Source: CAD feature listing. Evaluate the final solid. Frame: model axes, mm. Face numbers are marked on the shaded views. A direction names the side the tool comes from. Round coordinates to 2 decimals unless told otherwise and drop trailing zeros. Order: outer loops, then holes, each group sorted by start corner. A loop starts at its lowest first (then second) coordinate and runs counter-clockwise, first axis right, second up.
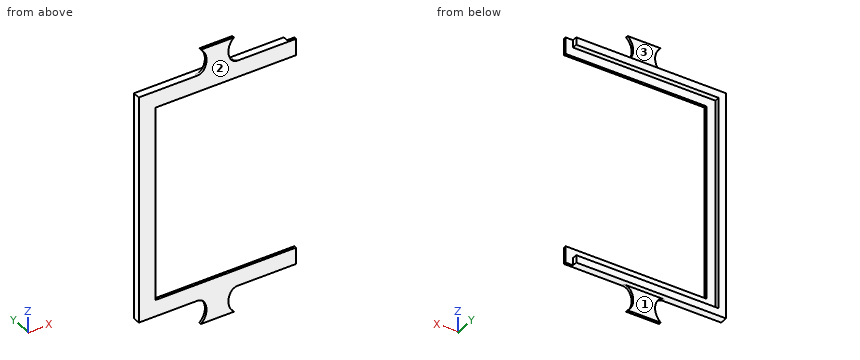
```python
from build123d import *

# Parameters (mm, degrees)
SKETCH1_W           = 10
SKETCH1_H           = 117.5
BOSS_EXTRUDE1_DEPTH = 1.5
BOSS_EXTRUDE2_DEPTH = 3


with BuildPart() as part:
    # Sketch1 → Boss-Extrude1 (new body)
    with BuildSketch(Plane(origin=(0, 0, 0), x_dir=(1, 0, 0), z_dir=(0, 1, 0))):
        with BuildLine():
            ThreePointArc((-7.95412424, -71.25), (-9.784251259, -69.419872981), (-12.284251259, -68.75))
            Line((-12.284251259, -68.75), (-47.65, -68.75))
            Line((-47.65, -68.75), (-47.65, -58.75))
            Line((-47.65, -58.75), (47.65, -58.75))
            Line((47.65, -58.75), (47.65, -68.75))
            Line((47.65, -68.75), (12.284251259, -68.75))
            ThreePointArc((12.284251259, -68.75), (9.784251259, -69.419872981), (7.95412424, -71.25))
            ThreePointArc((7.95412424, -71.25), (6.745685452, -77.865209555), (10, -83.75))
            Line((10, -83.75), (-10, -83.75))
            ThreePointArc((-10, -83.75), (-6.745685452, -77.865209555), (-7.95412424, -71.25))
        make_face()
        with Locations((-42.65, 0)):
            Rectangle(SKETCH1_W, SKETCH1_H)
        with BuildLine():
            ThreePointArc((-7.95412424, 71.25), (-6.745685452, 77.865209555), (-10, 83.75))
            Line((-10, 83.75), (10, 83.75))
            ThreePointArc((10, 83.75), (6.745685452, 77.865209555), (7.95412424, 71.25))
            ThreePointArc((7.95412424, 71.25), (9.784251259, 69.419872981), (12.284251259, 68.75))
            Line((12.284251259, 68.75), (47.65, 68.75))
            Line((47.65, 68.75), (47.65, 58.75))
            Line((47.65, 58.75), (-47.65, 58.75))
            Line((-47.65, 58.75), (-47.65, 68.75))
            Line((-47.65, 68.75), (-12.284251259, 68.75))
            ThreePointArc((-12.284251259, 68.75), (-9.784251259, 69.419872981), (-7.95412424, 71.25))
        make_face()
    extrude(amount=BOSS_EXTRUDE1_DEPTH)

    # Sketch2 → Boss-Extrude2 (add)
    with BuildSketch(Plane(origin=(0, 1.5, 0), x_dir=(1, 0, 0), z_dir=(0, 1, 0))):
        Polygon((-43.15, 64.25), (43.15, 64.25), (43.15, 68.75), (12.284251259, 68.75), (-12.284251259, 68.75), (-47.65, 68.75), (-47.65, -68.75), (-12.284251259, -68.75), (12.284251259, -68.75), (43.15, -68.75), (43.15, -64.25), (-43.15, -64.25), align=None)
    extrude(amount=BOSS_EXTRUDE2_DEPTH)


solid = part.part
```
1. Section C-C on y = 3.3. Return loops of the section in (x, z), plus the area to 3 significant figures.
2. First-contact query: pin 1 (2.5 mm diameter, centred on x = -16.5, y = 3, fed in from -Z); pin 2 (0.9 mm diameter, centred on y = 3, z = -67, fed in from +X); pin 3 (7.5 mm diameter, centred on x = -6, z = 75, fed in from +Y); pin 4 (6 mm diameter, centred on x = -33.5, z = -3.5, fed in from -Y). Flat tips, straight axial feed; report the tip coordinate or a pass-through.
3. Access query for the marked faces 1, 2 and 3. Directions: +Z, -Z, +X, -X, +Y, -Y. A direction counts if a zero-diameter tool reaches every point of the face in a straight line with its end or side. Return the directions, or none.
4. Section D-D on x = 37.5. Return loops of the section in (y, z).
5. Section B-B on z = 62. Return loops of the section in (x, y), plus the area to 3 significant figures.
6. Section A-A on x = -0.5. Return loops of the section in (y, z).
7. Line query: line 1 along Z through (x, y) = (22, 0.3); line 2 along Z through (x, y) = (37, 3.5); line 3 along X through (y, z) = (0.3, -56.5). Output: solid intervals per line, ascending.
Result:
1. outline: (-47.65, -68.75) - (43.15, -68.75) - (43.15, -64.25) - (-43.15, -64.25) - (-43.15, 64.25) - (43.15, 64.25) - (43.15, 68.75) - (-47.65, 68.75) - close
1. area: 1,400 mm2
2. pin 1: stops at z = -68.75
2. pin 2: stops at x = 43.15
2. pin 3: stops at y = 1.5
2. pin 4: passes through
3. face 1: -Z, +X, -X, +Y
3. face 2: +Z, -Z, +X, -X, -Y
3. face 3: +Z, +X, -X, +Y
4. outline: (0, -68.75) - (4.5, -68.75) - (4.5, -64.25) - (1.5, -64.25) - (1.5, -58.75) - (0, -58.75) - close; (0, 58.75) - (1.5, 58.75) - (1.5, 64.25) - (4.5, 64.25) - (4.5, 68.75) - (0, 68.75) - close
5. outline: (-47.65, 0) - (47.65, 0) - (47.65, 1.5) - (-43.15, 1.5) - (-43.15, 4.5) - (-47.65, 4.5) - close
5. area: 156 mm2
6. outline: (0, -83.75) - (1.5, -83.75) - (1.5, -68.75) - (4.5, -68.75) - (4.5, -64.25) - (1.5, -64.25) - (1.5, -58.75) - (0, -58.75) - close; (0, 58.75) - (1.5, 58.75) - (1.5, 64.25) - (4.5, 64.25) - (4.5, 68.75) - (1.5, 68.75) - (1.5, 83.75) - (0, 83.75) - close
7. line 1: z = -68.75 to -58.75, 58.75 to 68.75
7. line 2: z = -68.75 to -64.25, 64.25 to 68.75
7. line 3: x = -47.65 to -37.65
